Could you check a few things on this model? Use its own coordinates, in mm. Give positions to 0.01 mm unless a question says otherwise; leave off trailing zeros. Order: outer loops, then holes, each group sorted by start corner. A loop starts at its lowest first (then second) coordinate and runs counter-clockwise, first axis right, second up.
Autodesk Inventor part; units mm, degrees
ref_plane "YZ Plane" through (0, 0, 0) normal (1, 0, 0) x (0, 1, 0)
ref_plane "XZ Plane" through (0, 0, 0) normal (0, 1, 0) x (-1, 0, 0)
ref_plane "XY Plane" through (0, 0, 0) normal (0, 0, 1) x (1, 0, 0)
sketch "スケッチ1" plane through (0, 0, 0) normal (0, 1, 0) x (-1, 0, 0)
  circle A0 centre (0, 0) radius 3.15
  dimension "d0" = 6.3
extrude "押し出し1" add sketch "スケッチ1" along normal blind 1.5
sketch "スケッチ2" plane through (0, 0, 0) normal (0, -1, 0) x (1, 0, 0)
  circle A0 centre (0, 0) radius 2.1
  dimension "d3" = 4.2
extrude "押し出し2" add sketch "スケッチ2" along normal blind 1.38
sketch "スケッチ3" plane through (0, 1.5, 0) normal (0, 1, 0) x (1, 0, 0)
  point P0 (0, 0)
  point P1 (0, 0)
hole "穴1" at (0, 1.5, 0) direction (0, -1, 0) diameter 3 end through all
thread "ねじ1"
fillet "フィレット1" radius 0.3 1 edges at (3.15, 1.5, 0)
fillet "フィレット1" radius 0.1 1 edges at (3.15, 0, 0)
sketch "スケッチ4" plane through (0, 0, 0) normal (1, 0, 0) x (0, 1, 0)
  line L0 (-1.38, 2.1) -> (-1.38, -2.1)
  line L1 (-1.38, 2.1) -> (-0.58, 1.9)
  line L2 (-0.58, 1.9) -> (-0.58, 2.1)
  line L3 (-0.58, 2.1) -> (-1.38, 2.1)
  line L4 (-1.956, 0) -> (2.076, 0)
  point P0 (0, 0)
  dimension "d17" = 0.8
  dimension "d18" = 0.2
revolve "回転1" cut sketch "スケッチ4" angle 360 about axis through (0, -10, 0) along (0, 1, 0)
properties part number "ClinchingNut_M3T1.5_Slab1.4"
Item 1: Imagine slicing it at C-C on y = 0.5. List the corners of the cut face in (x, z) for me, then the cut area to 3 significant figures.
Findings:
outline: circle Ø6.3 at (0, 0); hole circle Ø3 at (0, 0)
area: 24.1 mm2
Item 2: For pin 1 (2.5 mm diameter, centred on x = 0, z = 0, fed in from -Y); pin 2 (1 mm diameter, centred on y = 1, z = 1.5, fed in from +X), each with a flat end and sliding along its axis, tell me the tip position at first contact or that it passes through.
Findings:
pin 1: passes through
pin 2: stops at x = 2.99
Item 3: We'd pull the mould along Z, two halves only. Please class faces 1 (the flat face through (1.4, -1.38, -0.9)), 2 (the cylindrical face through (-0.07, 0.04, -1.5)), 3 (the cylindrical face through (2.003, -0.286, -0.631)): +Z half, -Z half, draft (parallel to the pull), parting line (faces both ways), or undercut.
Findings:
face 1: draft
face 2: undercut
face 3: parting line
Item 4: Imagine slicing it at B-B on z = 0. List the corners of the cut face in (x, y) for me, then the cut area to 3 significant figures.
Findings:
outline: (-3.15, 0.1) arc R0.1 ccw to (-3.05, 0) - (-2.1, 0) - (-2.1, -0.58) - (-1.9, -0.58) - (-2.1, -1.38) - (-1.5, -1.38) - (-1.5, 1.5) - (-2.85, 1.5) arc R0.3 ccw to (-3.15, 1.2) - close; (1.5, -1.38) - (2.1, -1.38) - (1.9, -0.58) - (2.1, -0.58) - (2.1, 0) - (3.05, 0) arc R0.1 ccw to (3.15, 0.1) - (3.15, 1.2) arc R0.3 ccw to (2.85, 1.5) - (1.5, 1.5) - close
area: 6.40 mm2
Item 5: Please list where these lines run through material, in increasing order: line 1 along Z through (x, y) = (0, 0.4); line 2 along X through (y, z) = (-0.65, 0); line 3 along Y through (x, z) = (2, -1.5).
Findings:
line 1: z = -3.15 to -1.5, 1.5 to 3.15
line 2: x = -1.92 to -1.5, 1.5 to 1.92
line 3: y = 0 to 1.5
Item 6: Imagine slicing it at A-A on x = 0. List the corners of the cut face in (y, z) for me, then the cut area to 3 significant figures.
Findings:
outline: (-1.38, -2.1) - (-0.58, -1.9) - (-0.58, -2.1) - (0, -2.1) - (0, -3.05) arc R0.1 ccw to (0.1, -3.15) - (1.2, -3.15) arc R0.3 ccw to (1.5, -2.85) - (1.5, -1.5) - (-1.38, -1.5) - close; (-1.38, 1.5) - (1.5, 1.5) - (1.5, 2.85) arc R0.3 ccw to (1.2, 3.15) - (0.1, 3.15) arc R0.1 ccw to (0, 3.05) - (0, 2.1) - (-0.58, 2.1) - (-0.58, 1.9) - (-1.38, 2.1) - close
area: 6.40 mm2
Item 7: Imagine slicing it at D-D on y = -1.05. List the corners of the cut face in (x, z) for me (1 decimal).
Findings:
outline: circle Ø4 at (0, 0); hole circle Ø3 at (0, 0)
